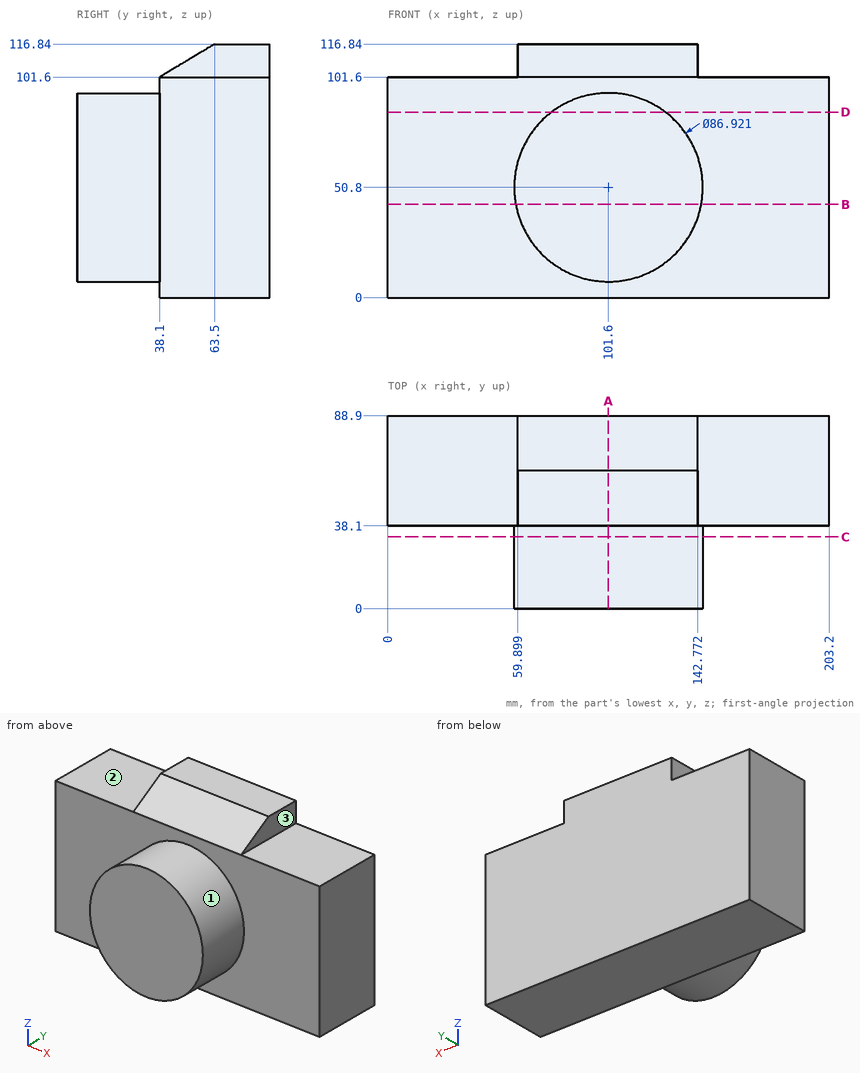
Source: three-view drawing plus pictorial views. Frame: mm from the lowest corner of the part. A direction names the side the tool comes from. Round coordinates to 2 decimals unless told otherwise and drop trailing zeros. Loops run counter-clockwise (first coordinate to the right, second up) from the corner with the lowest first, then second, coordinate; pieces in that order, holes last. Notation, with made-up numbers: M 46,-10 L 52,-10 A27 ccw 52,10 Z; hole C -30,61.25 d4. An arc over 180 degrees is marked long. Answer as CSV lines item,"result".
Q1. Cut plane C-C (y = 33). Return the cut outline in (x, z).
Verdict:
outline,"C 101.6,50.8 d86.92"
Q2. Line query: line 1 along Y through (x, z) = (123, 8.5); line 2 along Z through (x, y) = (34, 53); line 3 along Y through (x, z) = (87, 104.5) (1 decimal). Output: solid intervals per line, ascending.
Verdict:
line 1,"y = 38.1 to 88.9"
line 2,"z = 0 to 101.6"
line 3,"y = 42.9 to 88.9"
Q3. Reachability of the marked faces 1, 2 and 3 from +Z, -Z, +X, -X, +Y, -Y: full face, straight path, thin tool, end or side. Return the list, or none.
Verdict:
face 1,"-Y"
face 2,"+Z, -X, +Y, -Y"
face 3,"+Z, +X, +Y, -Y"
Q4. Cut plane D-D (z = 85.5). Return the cut outline in (x, y), plus the area to 3 significant figures.
Verdict:
outline,"M 0,38.1 L 75.43,38.1 L 75.43,0 L 127.77,0 L 127.77,38.1 L 203.2,38.1 L 203.2,88.9 L 0,88.9 Z"
area,"12,300 mm^2"
Q5. Cut plane B-B (z = 43). Return the cut outline in (x, y) (1 decimal), plus the area to 3 significant figures.
Verdict:
outline,"M 0,38.1 L 58.8,38.1 L 58.8,0 L 144.4,0 L 144.4,38.1 L 203.2,38.1 L 203.2,88.9 L 0,88.9 Z"
area,"13,600 mm^2"
Q6. Contact query for flat-ended pins moving along their axis: pin 1 (7.5 mm diameter, centred on y = 68.5, z = 106, fed in from -X); pin 2 (6 mm diameter, centred on y = 31, z = 89.5, fed in from +X) (1 decimal); pin 3 (5 mm diameter, centred on x = 154, y = 64.5, fed in from +Z). Output: stop coordinate, or through.
Verdict:
pin 1,"stops at x = 59.9"
pin 2,"stops at x = 126.4"
pin 3,"stops at z = 101.6"
Q7. Cut plane A-A (x = 101.6). Return the cut outline in (y, z).
Verdict:
outline,"M 0,7.34 L 38.1,7.34 L 38.1,0 L 88.9,0 L 88.9,116.84 L 63.5,116.84 L 38.1,101.6 L 38.1,94.26 L 0,94.26 Z"
